from build123d import *

# Parameters (mm, degrees)
SKETCH_1_W          = 80
SKETCH_1_H          = 50
SKETCH_1_W_2        = 30
SKETCH_1_H_2        = 29
EXTRUDE_1_DEPTH     = 2
SKETCH_5_W          = 2
SKETCH_5_H          = 50
EXTRUDE_2_DEPTH     = 2
SKETCH_2_W          = 30
SKETCH_2_H          = 4
CUT_EXTRUDE_1_DEPTH = 49.918299235
SKETCH_3_R          = 1.6
CUT_EXTRUDE_2_DEPTH = 49.918299235
SKETCH_6_W          = 1.5
SKETCH_6_H          = 4
CUT_EXTRUDE_4_DEPTH = 49.918299235
SKETCH_7_W          = 1.5
SKETCH_7_H          = 4
EXTRUDE_3_DEPTH     = 2
SKETCH_8_R          = 1.65
CUT_EXTRUDE_5_DEPTH = 49.918299235


with BuildPart() as part:
    # 草图1 → 凸台-拉伸1 (new body)
    with BuildSketch(Plane.XY):
        Rectangle(SKETCH_1_W, SKETCH_1_H)
        with Locations((0, 1.5)):
            Rectangle(SKETCH_1_W_2, SKETCH_1_H_2, mode=Mode.SUBTRACT)
    extrude(amount=EXTRUDE_1_DEPTH)

    # 草图5 → 凸台-拉伸2 (add)
    with BuildSketch(Plane.XY.offset(2)):
        with Locations((-41, 0)):
            Rectangle(SKETCH_5_W, SKETCH_5_H)
    extrude(amount=-EXTRUDE_2_DEPTH)

    # 草图2 → 切除-拉伸1 (cut, through all)
    with BuildSketch(Plane.XY.offset(2)):
        with Locations((0, -23)):
            Rectangle(SKETCH_2_W, SKETCH_2_H)
    extrude(amount=-CUT_EXTRUDE_1_DEPTH, mode=Mode.SUBTRACT)

    # 草图3 → 切除-拉伸2 (cut, through all)
    with BuildSketch(Plane.XY.offset(2)):
        with Locations((-39, -22)):
            Circle(SKETCH_3_R)
        with Locations((-19, -22)):
            Circle(SKETCH_3_R)
        with Locations(Location((17, -22, 0), (0, 0, 180))):
            Circle(SKETCH_3_R)
        with Locations(Location((37, -22, 0), (0, 0, 180))):
            Circle(SKETCH_3_R)
    extrude(amount=-CUT_EXTRUDE_2_DEPTH, mode=Mode.SUBTRACT)

    # 草图6 → 切除-拉伸4 (cut, through all)
    with BuildSketch(Plane.XY.offset(2)):
        with Locations((-15.75, -23)):
            Rectangle(SKETCH_6_W, SKETCH_6_H)
    extrude(amount=-CUT_EXTRUDE_4_DEPTH, mode=Mode.SUBTRACT)

    # 草图7 → 凸台-拉伸3 (add)
    with BuildSketch(Plane.XY.offset(2)):
        with Locations((14.25, -23)):
            Rectangle(SKETCH_7_W, SKETCH_7_H)
    extrude(amount=-EXTRUDE_3_DEPTH)

    # 草图8 → 切除-拉伸5 (cut, through all)
    with BuildSketch(Plane.XY.offset(2)):
        with Locations((-25, 11.5)):
            Circle(SKETCH_8_R)
        with Locations(Location((25, 11.5, 0), (0, 0, 180))):
            Circle(SKETCH_8_R)
        with Locations(Location((-25, -8.5, 0), (0, 0, 180))):
            Circle(SKETCH_8_R)
        with Locations((25, -8.5)):
            Circle(SKETCH_8_R)
    extrude(amount=-CUT_EXTRUDE_5_DEPTH, mode=Mode.SUBTRACT)


solid = part.part
Geometry: final body of the model. Coordinates: model frame, mm. A direction names the side the tool comes from. Give positions to 0.01 mm unless a question says otherwise; leave off trailing zeros. Loops run counter-clockwise (first coordinate to the right, second up) from the corner with the lowest first, then second, coordinate; pieces in that order, holes last. Notation, with made-up numbers: (46.5, -35) - (54.5, -35) arc R15 ccw to (54.5, -29) - close; hole circle Ø9 at (58.25, 66). An arc over 180 degrees is marked (long way). One line per question, with ' | ' between items. Start each with the question number.
(1) Section query B-B on z = 1.55. Count the separate pieces of the cut face and the enclosed holes in it, then the cut area to 3 significant figures.
(2) Section query D-D on x = -19. Return loops of the section in (y, z), then the cut area to 3 significant figures.
(3) Section query A-A on y = -8.5. Return loops of the section in (x, z).
(4) Contact query for a flat-ended pin moving along its axis: pin 1 (0.6 mm diameter, centred on x = 1, z = 1.5, fed in from -Y). Output: stop coordinate, or through.
(5) Ray query, line 1 (Y direction, x = -25, z = 1.35); line 2 (Y direction, x = -6, z = 1.55); line 3 (X direction, y = 12.5, z = 1.15). Return the intervals inside material, ascending. Write a range as from..to.
(6) Section query C-C on y = -22. Return loops of the section in (x, z).
(7) Pull-direction query (Y, two-part tool) for faces 1 (the cylindrical face through (-39.208, -20.414, 1.014)), 2 (the flat face through (-16.5, -23, 1)), 3 (the flat face through (0, 16, 1)), 4 (the flat face through (-2, 25, 1)); classes: released by +Y, released by -Y, zero draft, split by the parting line, or undercut.
(8) Reachability of faces 5 (the flat face through (-15, 1, 1)), 6 (the flat face through (-2, -21, 1)), 7 (the flat face through (-42, 0, 1)) from +Z, -Z, +X, -X, +Y, -Y: full face, straight path, thin tool, end or side. Return the list, or none.
The answers:
1) separate pieces: 1 | enclosed holes: 9 | area: 3,040 mm2
2) outline: (-25, 0) - (-23.6, 0) - (-23.6, 2) - (-25, 2) - close; (-20.4, 0) - (25, 0) - (25, 2) - (-20.4, 2) - close | area: 93.6 mm2
3) outline: (-42, 0) - (-26.65, 0) - (-26.65, 2) - (-42, 2) - close; (-23.35, 0) - (-15, 0) - (-15, 2) - (-23.35, 2) - close; (15, 0) - (23.35, 0) - (23.35, 2) - (15, 2) - close; (26.65, 0) - (40, 0) - (40, 2) - (26.65, 2) - close
4) pin 1: y = -21
5) line 1: -25..-10.15, -6.85..9.85, 13.15..25 | line 2: -21..-13, 16..25 | line 3: -42..-26.31, -23.69..-15, 15..23.69, 26.31..40
6) outline: (-42, 0) - (-40.6, 0) - (-40.6, 2) - (-42, 2) - close; (-37.4, 0) - (-20.6, 0) - (-20.6, 2) - (-37.4, 2) - close; (-17.4, 0) - (-16.5, 0) - (-16.5, 2) - (-17.4, 2) - close; (13.5, 0) - (15.4, 0) - (15.4, 2) - (13.5, 2) - close; (18.6, 0) - (35.4, 0) - (35.4, 2) - (18.6, 2) - close; (38.6, 0) - (40, 0) - (40, 2) - (38.6, 2) - close
7) face 1: undercut | face 2: zero draft | face 3: undercut | face 4: released by +Y
8) face 5: +Z, -Z | face 6: +Z, -Z, -Y | face 7: +Z, -Z, -X, +Y, -Y
